```python
from build123d import *

# Parameters (mm, degrees)
SKETCH1_R          = 1.25
EXTRUDE1_DEPTH     = 3
SKETCH2_R          = 1.25
EXTRUDE2_DEPTH     = 3
EXTRUDE4_DEPTH     = 1
CUT_EXTRUDE1_REACH = 15
SKETCH6_R          = 0.75


with BuildPart() as part:
    # Sketch1 → Extrude1 (new body)
    with BuildSketch(Plane(origin=(0, 0, 0), x_dir=(0, 0, -1), z_dir=(1, 0, 0))):
        with BuildLine():
            Line((4, 30), (4, 15.5))
            Line((4, 15.5), (-4, 3))
            Line((-4, 3), (-4, 0))
            Line((-4, 0), (-20, 0))
            Line((-20, 0), (-20, 3))
            Line((-20, 3), (-4, 28))
            Line((-4, 28), (-4, 30))
            ThreePointArc((-4, 30), (0, 34), (4, 30))
        make_face()
        with Locations((0, 15)):
            Circle(SKETCH1_R, mode=Mode.SUBTRACT)
        with Locations((0, 20)):
            Circle(SKETCH1_R, mode=Mode.SUBTRACT)
        with Locations((0, 25)):
            Circle(SKETCH1_R, mode=Mode.SUBTRACT)
        with Locations((0, 30)):
            Circle(SKETCH1_R, mode=Mode.SUBTRACT)
    extrude(amount=-EXTRUDE1_DEPTH)

    # Sketch2 → Extrude2 (add)
    with BuildSketch(Plane.XZ):
        with BuildLine():
            Line((-3, 20), (-11.5, 20))
            ThreePointArc((-11.5, 20), (-12.560660172, 19.560660172), (-13, 18.5))
            Line((-13, 18.5), (-13, 5.5))
            ThreePointArc((-13, 5.5), (-12.560660172, 4.439339828), (-11.5, 4))
            Line((-11.5, 4), (-3, 4))
            Line((-3, 4), (-3, 20))
        make_face()
        with Locations(Location((-8, 16, 0), (0, 0, 270))):  # turned: the seam where the file's is
            Circle(SKETCH2_R, mode=Mode.SUBTRACT)
        with Locations(Location((-8, 8, 0), (0, 0, 270))):  # turned: the seam where the file's is
            Circle(SKETCH2_R, mode=Mode.SUBTRACT)
    extrude(amount=-EXTRUDE2_DEPTH)

    # Sketch5 → Extrude4 (add, symmetric)
    with BuildSketch(Plane.XY.offset(12)):
        Polygon((-3, 3), (-9, 3), (-3, 13), align=None)
    extrude(amount=EXTRUDE4_DEPTH, both=True)

    # Sketch6 → Cut-Extrude1 (cut, up to next)
    with BuildSketch(Plane(origin=(0, 0, 0), x_dir=(0, 0, -1), z_dir=(1, 0, 0)), mode=Mode.PRIVATE) as cut_extrude1_sk1:
        with Locations((-2.5, 12.5)):
            Circle(SKETCH6_R)
    cut_extrude1_tool1 = extrude(cut_extrude1_sk1.sketch, amount=-CUT_EXTRUDE1_REACH, mode=Mode.PRIVATE) & part.part
    add(cut_extrude1_tool1.solids().sort_by_distance((0, 12.5, 2.5))[0], mode=Mode.SUBTRACT)
    # Sketch6 → Cut-Extrude1 (cut, up to next)
    with BuildSketch(Plane(origin=(0, 0, 0), x_dir=(0, 0, -1), z_dir=(1, 0, 0)), mode=Mode.PRIVATE) as cut_extrude1_sk2:
        with Locations((-2.5, 22.5)):
            Circle(SKETCH6_R)
    cut_extrude1_tool2 = extrude(cut_extrude1_sk2.sketch, amount=-CUT_EXTRUDE1_REACH, mode=Mode.PRIVATE) & part.part
    add(cut_extrude1_tool2.solids().sort_by_distance((0, 22.5, 2.5))[0], mode=Mode.SUBTRACT)
    # Sketch6 → Cut-Extrude1 (cut, up to next)
    with BuildSketch(Plane(origin=(0, 0, 0), x_dir=(0, 0, -1), z_dir=(1, 0, 0)), mode=Mode.PRIVATE) as cut_extrude1_sk3:
        with Locations((-2.5, 17.5)):
            Circle(SKETCH6_R)
    cut_extrude1_tool3 = extrude(cut_extrude1_sk3.sketch, amount=-CUT_EXTRUDE1_REACH, mode=Mode.PRIVATE) & part.part
    add(cut_extrude1_tool3.solids().sort_by_distance((0, 17.5, 2.5))[0], mode=Mode.SUBTRACT)
    # Sketch6 → Cut-Extrude1 (cut, up to next)
    with BuildSketch(Plane(origin=(0, 0, 0), x_dir=(0, 0, -1), z_dir=(1, 0, 0)), mode=Mode.PRIVATE) as cut_extrude1_sk4:
        Polygon((0, 0), (0, 25), (-8, 25), (-8, 35), (7, 35), (7, 0), align=None)
    cut_extrude1_tool4 = extrude(cut_extrude1_sk4.sketch, amount=-CUT_EXTRUDE1_REACH, mode=Mode.PRIVATE) & part.part
    add(cut_extrude1_tool4.solids().sort_by_distance((0, 20.576923, -1.653846))[0], mode=Mode.SUBTRACT)


solid = part.part
```
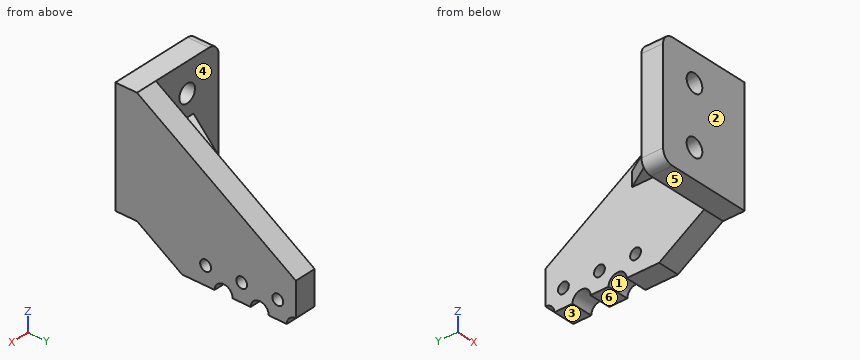
The model under review builds one solid part; all positions refer to its coordinate system, in mm. Face numbers are marked on the shaded views. A direction names the side the tool comes from. Round coordinates to 2 decimals unless told otherwise and drop trailing zeros. Order: outer loops, then holes, each group sorted by start corner. A loop starts at its lowest first (then second) coordinate and runs counter-clockwise, first axis right, second up. Notation, with made-up numbers: (20, 24.25) -> (38, 24.25) arc R18 cw to (38, 39.25) -> close; hole circle Ø7 at (68.25, 28.25). An arc over 180 degrees is marked (long way). One line per item, written item: value. Start each with the question number.
Q1. Wall thickness on line 1 (X direction, y = 1.15, z = 16); line 2 (Y direction, x = -0.9, z = 2.5); line 3 (X direction, y = 5.5, z = 4): over which ranges is each line inside the solid? List them lowest first.
Q2. Take a section at D-D (y = 6.5). Write out the cut boundary in (x, z).
Q3. Take a section at B-B (y = 17.5). Write out the cut boundary in (x, z).
Q4. Machinability: for the marked faces 4, 5 and 6, which of the approach directions +Z, -Z, +X, -X, +Y, -Y give a long, thin tool a straight path to every point of the face, cutting with its end or side? Answer none if there is none.
Q5. Take a section at A-A (z = 8). Write out the cut boundary in (x, y).
Q6. Mouldability with a two-part tool opening along Y and no side actions: class the marked faces 1, 2 and 3 as released by +Y, released by -Y, zero draft, split by the parting line, or undercut.
Q7. Take a section at C-C (x = -5.25). Write out the cut boundary in (y, z), and give its area (3 significant figures).
Q8. Clearance check with flat-ended pins moving along their axes: pin 1 Ø4 at (x, z) = (-8, 16) entering from -Y; pin 2 Ø3 at (x, z) = (-6.5, 15.5) entering from +Y; pin 3 Ø5 at (x, y) = (-6.5, 8.5) entering from +Z; pin 4 Ø2.5 at (y, z) = (22.5, 2.5) entering from -X. State where each tip first meets the part, or that it passes through.
Reported:
1. line 1: x = -13 to -9.25, -6.75 to 0
1. line 2: y = 5.34 to 11.75, 13.25 to 16.75, 18.25 to 21.75, 23.25 to 25
1. line 3: x = -3 to 0
2. outline: (-6.9, 11) -> (-3, 11) -> (-3, 1.76) -> (0, 1.76) -> (0, 17.76) -> (-3, 17.76) -> (-3, 13) -> (-6.9, 13) -> close
3. outline: (-3, 0) -> (0, 0) -> (0, 1.75) -> (-3, 1.75) -> close; (-3, 3.25) -> (0, 3.25) -> (0, 10.72) -> (-3, 10.72) -> close
4. face 4: -X, +Y
4. face 5: -Z, +X, -X, -Y
4. face 6: -Z, +X, -X, +Y, -Y
5. outline: (-13, 0) -> (-9.25, 0) -> (-9.25, 3) -> (-13, 3) -> close; (-6.75, 0) -> (0, 0) -> (0, 21.75) -> (-3, 21.75) -> (-3, 3) -> (-6.75, 3) -> close
6. face 1: undercut
6. face 2: released by -Y
6. face 3: zero draft
7. outline: (0, 4) -> (3, 4) -> (3, 11) -> (9.25, 11) -> (9.25, 13) -> (3, 13) -> (3, 20) -> (0, 20) -> close
7. area: 60.5 mm2
8. pin 1: stops at y = 0
8. pin 2: stops at y = 3
8. pin 3: stops at z = 13
8. pin 4: stops at x = -3
